The figure shows three views and two pictorial views of one solid part (mm, origin at its lowest corner). Answer the questions. A direction names the side the tool comes from. Give positions to 0.01 mm unless a question says otherwise; leave off trailing zeros. Write each loop counter-clockwise with the first axis right and the second up, starting at its lowest first coordinate (ties: lowest second). Pieces come first, ordered by that corner, then holes. Notation, with made-up numbers: (58, -14.75) -> (64, -14.75) arc R12 cw to (64, -2.75) -> close; hole circle Ø5 at (52.25, -18). An arc over 180 degrees is marked (long way). Answer as CSV lines item,"result". Start each with the question number.
1. The part is cut by section C-C, the plane y = 20. Determine the outline of the cut face in (x, z), and give its area (3 significant figures).
2. A tool of negligible diameter and unlimited length cuts with its end or side. For the marked faces 4, 5 and 6, from which of +Z, -Z, +X, -X, +Y, -Y can it reach the whole face along a straight path? Write none if from no direction.
3. The part is cut by section D-D, the plane z = 19. Determine the outline of the cut face in (x, y).
4. The part is cut by section A-A, the plane y = 25. Determine the outline of the cut face in (x, z).
5. The part is cut by section B-B, the plane x = 11.25. Determine the outline of the cut face in (y, z).
6. Find the intervals of material crossed by line 1 (Y direction, x = 31.5, z = 12); line 2 (Z direction, x = 34.5, y = 3); line 3 (Y direction, x = 2, z = 46) (1 decimal), in increasing order.
7. For a pull along X with two mould halves and no side action, classify the marked faces 1, 2 and 3 as pulls with the +X half, pulls with the -X half, needs draft (parallel to the pull), parting line crosses it, or undercut.
8. Given pin 1 (2.5 mm diameter, centred on x = 35.15, z = 15.62, fed in from -Y); pin 2 (2 mm diameter, centred on y = 6.5, z = 23.5, fed in from +X); pin 3 (11.5 mm diameter, centred on x = 13.5, y = 30.5, fed in from -Z), each flat-ended and moving along its own axis, determine where each tip first touches the part or whether it passes through.
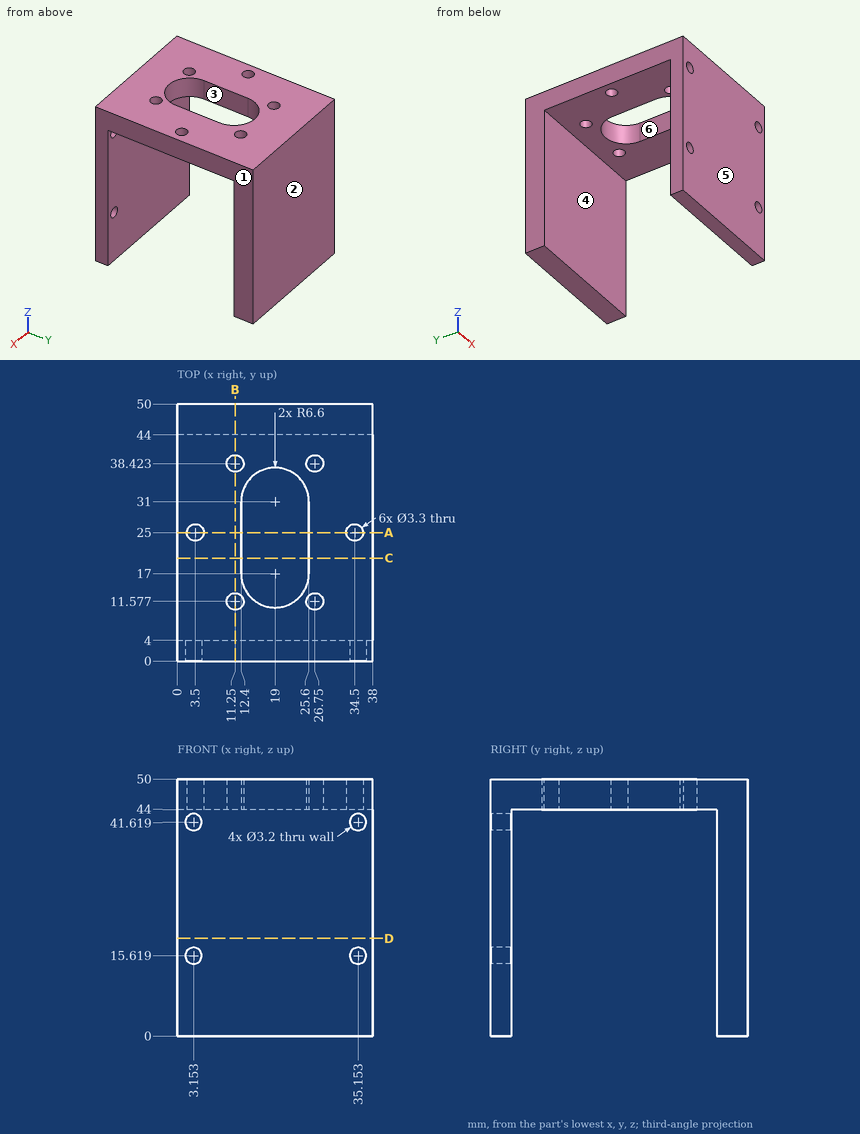
Results found:
1,outline,"(0, 44) -> (12.4, 44) -> (12.4, 50) -> (0, 50) -> close; (25.6, 44) -> (38, 44) -> (38, 50) -> (25.6, 50) -> close"
1,area,"149 mm²"
2,face 4,"-Z, +X, -X"
2,face 5,"+Z, -Z, +X, -X, -Y"
2,face 6,"+Z, -Z"
3,outline,"(0, 0) -> (38, 0) -> (38, 4) -> (0, 4) -> close; (0, 44) -> (38, 44) -> (38, 50) -> (0, 50) -> close"
4,outline,"(0, 44) -> (1.85, 44) -> (1.85, 50) -> (0, 50) -> close; (5.15, 44) -> (12.4, 44) -> (12.4, 50) -> (5.15, 50) -> close; (25.6, 44) -> (32.85, 44) -> (32.85, 50) -> (25.6, 50) -> close; (36.15, 44) -> (38, 44) -> (38, 50) -> (36.15, 50) -> close"
5,outline,"(0, 0) -> (4, 0) -> (4, 44) -> (9.93, 44) -> (9.93, 50) -> (0, 50) -> close; (13.23, 44) -> (36.77, 44) -> (36.77, 50) -> (13.23, 50) -> close; (40.07, 44) -> (44, 44) -> (44, 0) -> (50, 0) -> (50, 50) -> (40.07, 50) -> close"
6,line 1,"y = 0 to 4, 44 to 50"
6,line 2,"z = 0 to 14.16, 17.08 to 40.16, 43.08 to 50"
6,line 3,"y = 0 to 24.3, 25.7 to 50"
7,face 1,"pulls with the +X half"
7,face 2,"needs draft"
7,face 3,"undercut"
8,pin 1,"stops at y = 44"
8,pin 2,"passes through"
8,pin 3,"stops at z = 44"
